from build123d import *

# Parameters (mm, degrees)
F0_W     = 36.4
F0_H     = 71.8
F1_DEPTH = 8.5
F2_W     = 34
F2_H     = 65.6
F3_DEPTH = 6
F5_DEPTH = 6


with BuildPart() as f1:
    # F0 (on Top) → F1 (new body)
    with BuildSketch(Plane.XY):
        with Locations((18.2, 35.9)):
            Rectangle(F0_W, F0_H)
    extrude(amount=F1_DEPTH)

    # F2 (on face) → F3 (cut)
    with BuildSketch(Plane.XY.offset(8.5)):
        with Locations((18.2, 37.8)):
            Rectangle(F2_W, F2_H)
    extrude(amount=-F3_DEPTH, mode=Mode.SUBTRACT)

    # F4 (on face) → F5 (join)
    with BuildSketch(Plane.XY.offset(2.5)):
        Polygon((24.4, 70.6), (23.2, 70.6), (23.2, 62.257143), (13.2, 62.257143), (12, 62.257143), (1.2, 62.257143), (1.2, 61.057143), (12, 61.057143), (13.2, 61.057143), (23.2, 61.057143), (23.2, 52.714286), (13.2, 52.714286), (12, 52.714286), (1.2, 52.714286), (1.2, 51.514286), (12, 51.514286), (13.2, 51.514286), (23.2, 51.514286), (23.2, 43.171429), (13.2, 43.171429), (12, 43.171429), (1.2, 43.171429), (1.2, 41.971429), (12, 41.971429), (13.2, 41.971429), (23.2, 41.971429), (23.2, 33.628571), (13.2, 33.628571), (12, 33.628571), (1.2, 33.628571), (1.2, 32.428571), (12, 32.428571), (13.2, 32.428571), (23.2, 32.428571), (23.2, 24.085714), (13.2, 24.085714), (12, 24.085714), (1.2, 24.085714), (1.2, 22.885714), (12, 22.885714), (13.2, 22.885714), (23.2, 22.885714), (23.2, 14.542857), (13.2, 14.542857), (12, 14.542857), (1.2, 14.542857), (1.2, 13.342857), (12, 13.342857), (13.2, 13.342857), (23.2, 13.342857), (23.2, 5), (24.4, 5), (24.4, 13.342857), (35.2, 13.342857), (35.2, 14.542857), (24.4, 14.542857), (24.4, 22.885714), (35.2, 22.885714), (35.2, 24.085714), (24.4, 24.085714), (24.4, 32.428571), (35.2, 32.428571), (35.2, 33.628571), (24.4, 33.628571), (24.4, 41.971429), (35.2, 41.971429), (35.2, 43.171429), (24.4, 43.171429), (24.4, 51.514286), (35.2, 51.514286), (35.2, 52.714286), (24.4, 52.714286), (24.4, 61.057143), (35.2, 61.057143), (35.2, 62.257143), (24.4, 62.257143), align=None)
    extrude(amount=F5_DEPTH)


with BuildPart() as f6_1:
    # F6: copy of F1
    add(f1.part)


solid = f1.part
Source: CAD feature listing. Evaluate the final solid. Frame: model axes, mm. Give positions to 0.01 mm unless a question says otherwise; leave off trailing zeros. Write each loop counter-clockwise with the first axis right and the second up, starting at its lowest first coordinate (ties: lowest second). Pieces come first, ordered by that corner, then holes. Notation, with made-up numbers: M 44.5,-38.75 L 50.5,-38.75 A28 ccw 50.5,-10.75 Z; hole C 29.5,12.5 d9. An arc over 180 degrees is marked long. Return JSON: item names as keys, results as strings. Group by question number.
1) First-contact query: pin 1 Ø3 at (x, y) = (6, 47.5) entering from +Z. Flat tip, straight axial feed; report the tip coordinate or a pass-through.
2) Ray query, L1, parallel to X at y = 55, z = 4.5; L2, parallel to Z at x = 5, y = 59. Return the intervals inside material, ascending.
3) Draft query along X for faces 1 (the face through (12, 13.343, 5)), 2 (the face through (18, 36, 0)), 3 (the face through (36.4, 35, 4)). Return one class per face: released by +X, released by -X, zero draft, split by the parting line, or undercut.
4) Cut plane A-A, the plane y = 28.5. Output: boundary loops of the cut face in (x, z).
5) Cut plane C-C, the plane z = 6.75. Give the number of separate pieces and of enclosed holes in the cut face, then the cut area to 3 significant figures.
Data:
{
 "1": {"pin 1": "stops at z = 2.5"},
 "2": {"L1": "x = 0 to 1.2, 23.2 to 24.4, 35.2 to 36.4", "L2": "z = 0 to 2.5"},
 "3": {"face 1": "undercut", "face 2": "zero draft", "face 3": "released by +X"},
 "4": {"outline": "M 0,0 L 36.4,0 L 36.4,8.5 L 35.2,8.5 L 35.2,2.5 L 24.4,2.5 L 24.4,8.5 L 23.2,8.5 L 23.2,2.5 L 1.2,2.5 L 1.2,8.5 L 0,8.5 Z"},
 "5": {"separate pieces": "1", "enclosed holes": "14", "area": "698 mm²"}
}
